Part model, mm, in its own coordinate system. Round coordinates to 2 decimals unless told otherwise and drop trailing zeros. Loops run counter-clockwise (first coordinate to the right, second up) from the corner with the lowest first, then second, coordinate; pieces in that order, holes last.
(1) Cut at D-D on x = 17.5. List the corners of the cut face in (y, z).
(2) Flat gauge pins, fed straight in: pin 1 (2.5 mm diameter, centred on x = -42.5, z = 3, fed in from +Y); pin 2 (1.5 mm diameter, centred on x = -41.5, z = 1.5, fed in from -Y); pin 3 (3 mm diameter, centred on y = 53, z = 3.5, fed in from -X). Where does each tip first touch, or does it go through?
(3) Cut at B-B on y = 6. List the corners of the cut face in (x, z), then the cut area to 3 significant figures.
(4) Cut at A-A on x = 30. List the corners of the cut face in (y, z), then the cut area to 3 significant figures.
(5) Probe probe 1 along Y at (x, z) = (30, 3.5); probe 2 along X at (y, z) = (14, 4.15); probe 3 along X at (y, z) = (-11.5, 2.25). List the from-to ranges inside material, lowest first.
(6) Cut at C-C on z = 1.5. List the corners of the cut face in (x, y).
from build123d import *

# Parameters (mm, degrees)
BOSS_EXTRUDE1_DEPTH = 5
SKETCH2_W           = 29
SKETCH2_H           = 60
SKETCH2_W_2         = 20
SKETCH2_H_2         = 40
CUT_EXTRUDE1_DEPTH  = 5
SKETCH3_W           = 5
SKETCH3_H           = 15
BOSS_EXTRUDE2_DEPTH = 5
CUT_EXTRUDE2_DEPTH  = 5
SKETCH5_R           = 1.5
CUT_EXTRUDE3_DEPTH  = 5


with BuildPart() as part:
    # Sketch1 → Boss-Extrude1 (new body)
    with BuildSketch(Plane.XY):
        Polygon((0, 31.783783784), (10, 66.783783784), (40, 66.783783784), (40, 21.783783784), (40, -48.216216216), (-40, -48.216216216), (-40, 31.783783784), align=None)
    extrude(amount=BOSS_EXTRUDE1_DEPTH)

    # Sketch2 → Cut-Extrude1 (cut)
    with BuildSketch(Plane.XY.offset(5)):
        with Locations((-10.5, -8.216216216)):
            Rectangle(SKETCH2_W, SKETCH2_H)
        with Locations((25, 36.783783784)):
            Rectangle(SKETCH2_W_2, SKETCH2_H_2)
    extrude(amount=-CUT_EXTRUDE1_DEPTH, mode=Mode.SUBTRACT)

    # Sketch3 → Boss-Extrude2 (add)
    with BuildSketch(Plane.ZY.offset(40)):
        with Locations((2.5, 9.283783784)):
            Rectangle(SKETCH3_W, SKETCH3_H)
        with Locations((2.5, -25.716216216)):
            Rectangle(SKETCH3_W, SKETCH3_H)
    extrude(amount=BOSS_EXTRUDE2_DEPTH)

    # Sketch4 → Cut-Extrude2 (cut)
    with BuildSketch(Plane.XY.offset(5)):
        Polygon((-40, 31.783783784), (-25, 31.783783784), (-40, 24.283783784), align=None)
        Polygon((-40, -48.216216216), (-40, -40.716216216), (-25, -48.216216216), align=None)
    extrude(amount=-CUT_EXTRUDE2_DEPTH, mode=Mode.SUBTRACT)

    # Sketch5 → Cut-Extrude3 (cut)
    with BuildSketch(Plane.XY.offset(5)):
        with Locations((30, 1.783783784)):
            Circle(SKETCH5_R)
    extrude(amount=-CUT_EXTRUDE3_DEPTH, mode=Mode.SUBTRACT)


solid = part.part
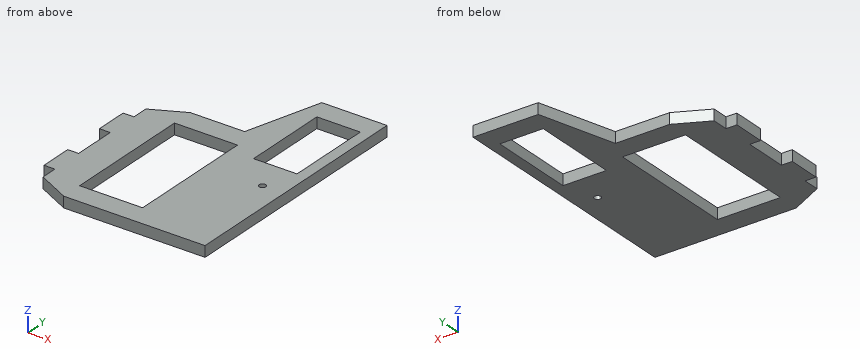
Final values:
1. outline: (-48.22, 0) - (16.78, 0) - (16.78, 5) - (-48.22, 5) - close; (56.78, 0) - (66.78, 0) - (66.78, 5) - (56.78, 5) - close
2. pin 1: stops at y = 16.78
2. pin 2: stops at y = -33.22
2. pin 3: stops at x = 5.63
3. outline: (-45, 0) - (-25, 0) - (-25, 5) - (-45, 5) - close; (4, 0) - (40, 0) - (40, 5) - (4, 5) - close
3. area: 280 mm2
4. outline: (-48.22, 0) - (0.28, 0) - (0.28, 5) - (-48.22, 5) - close; (3.28, 0) - (16.78, 0) - (16.78, 5) - (3.28, 5) - close; (56.78, 0) - (66.78, 0) - (66.78, 5) - (56.78, 5) - close
4. area: 360 mm2
5. probe 1: y = -48.22 to 0.28, 3.28 to 16.78, 56.78 to 66.78
5. probe 2: x = -45 to -25, 4 to 40
5. probe 3: x = -40 to -25, 4 to 40
6. outline: (-45, -33.22) - (-40, -33.22) - (-40, -40.72) - (-25, -48.22) - (40, -48.22) - (40, 66.78) - (10, 66.78) - (0, 31.78) - (-25, 31.78) - (-40, 24.28) - (-40, 16.78) - (-45, 16.78) - (-45, 1.78) - (-40, 1.78) - (-40, -18.22) - (-45, -18.22) - close; hole (-25, -38.22) - (4, -38.22) - (4, 21.78) - (-25, 21.78) - close; hole (15, 16.78) - (35, 16.78) - (35, 56.78) - (15, 56.78) - close; hole circle Ø3 at (30, 1.78)
